For this review, take the finished solid that the model builds, in its own axes (mm). A direction names the side the tool comes from. Round coordinates to 2 decimals unless told otherwise and drop trailing zeros. Order: outer loops, then holes, each group sorted by start corner. A loop starts at its lowest first (then second) coordinate and runs counter-clockwise, first axis right, second up.
from build123d import *

# Parameters (mm, degrees)
BOSS_EXTRUDE1_DEPTH                                 = 13
FILLET2_R                                           = 8
SKETCH2_R                                           = 1.7
CUT_EXTRUDE1_DEPTH                                  = 41
SKETCH3_R                                           = 3.5
CUT_EXTRUDE2_DEPTH                                  = 28
CSK_FOR_M3_COUNTERSUNK_FLAT_HEAD_SCREW1_D           = 3.2
CSK_FOR_M3_COUNTERSUNK_FLAT_HEAD_SCREW1_CSINK_D     = 6.3
CSK_FOR_M3_COUNTERSUNK_FLAT_HEAD_SCREW1_CSINK_ANGLE = 90
FILLET3_R                                           = 2


with BuildPart() as part:
    # Sketch1 → Boss-Extrude1 (new body)
    with BuildSketch(Plane(origin=(0, 0, 0), x_dir=(0, 0, -1), z_dir=(1, 0, 0))):
        Polygon((0, -16), (-16, -16), (0, 0), (-26, 0), (-26, 8), (6, 8), (6, -16), align=None)
    extrude(amount=BOSS_EXTRUDE1_DEPTH)

    # Fillet2
    fillet2_edges = [part.edges().sort_by_distance(p)[0] for p in [
        (6.5, 8, -6),
        (6.5, -16, -6),
    ]]
    fillet(fillet2_edges, radius=FILLET2_R)

    # Sketch2 → Cut-Extrude1 (cut)
    with BuildSketch(Plane(origin=(0, 0, -6), x_dir=(-1, 0, 0), z_dir=(0, 0, -1))):
        with Locations((-6.5, 4)):
            Circle(SKETCH2_R)
    extrude(amount=-CUT_EXTRUDE1_DEPTH, mode=Mode.SUBTRACT)

    # Sketch3 → Cut-Extrude2 (cut)
    with BuildSketch(Plane(origin=(0, 0, -6), x_dir=(-1, 0, 0), z_dir=(0, 0, -1))):
        with Locations((-6.5, 4)):
            Circle(SKETCH3_R)
    extrude(amount=-CUT_EXTRUDE2_DEPTH, mode=Mode.SUBTRACT)

    # CSK for M3 Countersunk Flat Head Screw1 (through all)
    with Locations(Plane(origin=(0, 0, 22), x_dir=(-1, 0, 0), z_dir=(0, 0, -1))):
        with Locations((-6.5, 4)):
            CounterSinkHole(CSK_FOR_M3_COUNTERSUNK_FLAT_HEAD_SCREW1_D / 2, CSK_FOR_M3_COUNTERSUNK_FLAT_HEAD_SCREW1_CSINK_D / 2, counter_sink_angle=CSK_FOR_M3_COUNTERSUNK_FLAT_HEAD_SCREW1_CSINK_ANGLE)

    # Fillet3
    fillet3_edges = [part.edges().sort_by_distance(p)[0] for p in [
        (6.5, 0, 0),
    ]]
    fillet(fillet3_edges, radius=FILLET3_R)


solid = part.part
(1) Add section A-A on z = 10. Give the boundary of the cut face in (x, y), plus the area to 3 significant figures.
(2) Draft analysis for pull direction Y (two halves, no side actions). For faces 3 (the face through (13, 2, 6)), 4 (the face through (6, 8, 14)), 5 (the face through (6.591, -1.204, 2.994)), 6 (the face through (7.259, 0.583, 7.812)), state which applies: pulls with the +Y half, pulls with the -Y half, needs draft (parallel to the pull), parting line crosses it, or undercut.
(3) Add section C-C on y = 4. Give the boundary of the cut face in (x, z), plus the area to 3 significant figures.
(4) Add section D-D on x = 6.5. Give the boundary of the cut face in (y, z).
(5) Add section B-B on x = 1. Give the boundary of the cut face in (y, z).
(6) Wall thickness on L1, parallel to X at y = 4, z = 10.25; L2, parallel to Y at x = 6.5, z = 25.2; L3, parallel to X at y = 4, z = 25: over which ranges is each line inside the solid? List them lowest first.
(7) Clearance check with flat-ended pins moving along their axes: P1, Ø3, axis at x = 2, y = 0.5, coming from the -Z side; P2, Ø3.5, axis at x = 6.5, y = 4, coming from the -Z side; P3, Ø4, axis at x = 9, z = 20, coming from the -Y side. State where each tip first meets the part, or that it passes through.
(8) Tool access review of faces 1 (the face through (6, -10, 10)), 2 (the face through (6.87, 2.34, 24.71)): name each direction out of +Z, -Z, +X, -X, +Y, -Y from which nothing blocks a thin tool from reaching the whole face with its end or side.
Here are the results:
1. outline: (0, -16) - (13, -16) - (13, -10) - (0, -10) - close; (0, 0) - (13, 0) - (13, 8) - (0, 8) - close; hole circle Ø7 at (6.5, 4)
1. area: 144 mm2
2. face 3: needs draft
2. face 4: pulls with the +Y half
2. face 5: undercut
2. face 6: undercut
3. outline: (0, -4.93) - (3, -4.93) - (3, 22) - (3.35, 22) - (4.8, 23.45) - (4.8, 26) - (0, 26) - close; (8.2, 23.45) - (9.65, 22) - (10, 22) - (10, -4.93) - (13, -4.93) - (13, 26) - (8.2, 26) - close
3. area: 198 mm2
4. outline: (-16, 2) arc R8 ccw to (-8, -6) - (0, -6) arc R8 ccw to (0.5, -5.98) - (0.5, 22) - (0.85, 22) - (2.3, 23.45) - (2.3, 26) - (0, 26) - (0, 4.83) arc R2 cw to (-3.41, 3.41) - (-16, 16) - close; (5.7, 23.45) - (7.15, 22) - (7.5, 22) - (7.5, -0.78) arc R8 ccw to (8, 2) - (8, 26) - (5.7, 26) - close
5. outline: (-16, 2) arc R8 ccw to (-8, -6) - (0, -6) arc R8 ccw to (8, 2) - (8, 26) - (0, 26) - (0, 4.83) arc R2 cw to (-3.41, 3.41) - (-16, 16) - close
6. L1: x = 0 to 3, 10 to 13
6. L2: y = 0 to 2.3, 5.7 to 8
6. L3: x = 0 to 4.8, 8.2 to 13
7. P1: stops at z = -6
7. P2: stops at z = 23.4
7. P3: stops at y = 0
8. face 1: +Z, +X, -X
8. face 2: +Z, -Z
